```python
from build123d import *

# Parameters (mm, degrees)
SKETCH1_R           = 2.1
BOSS_EXTRUDE1_DEPTH = 360


with BuildPart() as part:
    # Sketch1 (on Front Plane) → Boss-Extrude1 (new body)
    with BuildSketch(Plane.XY):
        Polygon((-5.074586208, 10), (-3.28215401, 8.207567802), (-5.525872647, 8.207567802), (-5.525872647, 6.527957213), (-2.897129144, 3.89921371), (2.868055105, 3.89921371), (5.496798608, 6.527957213), (5.496798608, 8.207567802), (3.093698324, 8.207567802), (4.886130522, 10), (10, 10), (10, 4.886130522), (8.207567802, 3.093698324), (8.207567802, 5.496798608), (6.527957213, 5.496798608), (3.89921371, 2.868055105), (3.89921371, -2.897129144), (6.527957213, -5.525872647), (8.207567802, -5.525872647), (8.207567802, -3.28215401), (10, -5.074586208), (10, -10), (5.074586208, -10), (3.28215401, -8.207567802), (5.525872647, -8.207567802), (5.525872647, -6.527957213), (2.897129144, -3.89921371), (-2.868055105, -3.89921371), (-5.496798608, -6.527957213), (-5.496798608, -8.207567802), (-3.093698324, -8.207567802), (-4.886130522, -10), (-10, -10), (-10, -4.886130522), (-8.207567802, -3.093698324), (-8.207567802, -5.496798608), (-6.527957213, -5.496798608), (-3.89921371, -2.868055105), (-3.89921371, 2.897129144), (-6.527957213, 5.525872647), (-8.207567802, 5.525872647), (-8.207567802, 3.28215401), (-10, 5.074586208), (-10, 10), align=None)
        with Locations(Location((0, 0, 0), (0, 0, 180))):
            Circle(SKETCH1_R, mode=Mode.SUBTRACT)
    extrude(amount=BOSS_EXTRUDE1_DEPTH)


solid = part.part
```
Geometry check sheet. Reference: the model listing, model coordinates, mm. A direction names the side the tool comes from. Give positions to 0.01 mm unless a question says otherwise; leave off trailing zeros. Write item = value, one per line.
(1) Material ranges on line 1 (Y direction, x = -0.5, z = 202); line 2 (X direction, y = 7.25, z = 92.5); line 3 (Y direction, x = -8.25, z = 263), recorded low to high. Write a range as [from, to].
Answer below:
line_1 = [-3.9, -2.04], [2.04, 3.9]
line_2 = [-10, -5.53], [5.5, 10]
line_3 = [-10, -3.14], [3.32, 10]
(2) Release check for a two-part mould opening along Y. For faces 1 (the face through (3.899, 0, 177)), 2 (the face through (-3.899, 0, 177)), 3 (the face through (0, -3.899, 177)), 4 (the face through (0.1, 2.4, 0)) record: released by +Y, released by -Y, zero draft, split by the parting line, or undercut.
Answer below:
face_1 = undercut
face_2 = undercut
face_3 = released by -Y
face_4 = zero draft
(3) Tool access check on faces 5 (the face through (0, 3.899, 177)), 6 (the face through (0.1, 2.4, 360)). Record the directions out of +Z, -Z, +X, -X, +Y, -Y that give a thin tool (end or side, any length) a straight path to the whole face; none if there is none.
Answer below:
face_5 = +Z, -Z, +Y
face_6 = +Z, +X, -X, +Y, -Y
(4) Gauge pin test, flat ends, axial feed: pin 1 Ø0.7 at (y, z) = (-4.5, 139.5) entering from -X; pin 2 Ø1.7 at (y, z) = (1, 264) entering from +X; pin 3 Ø1.5 at (x, y) = (-6.5, -1.5) entering from +Z (3 decimals); pin 4 Ø4.5 at (x, z) = (0.5, 114.5) entering from +Y. Record the tip position at first contact, or that the pin passes through.
Answer below:
pin_1 = -9.96
pin_2 = 3.9
pin_3 = through
pin_4 = 3.9
